Input: part model. Units: mm. Frame: model coordinates. A direction names the side the tool comes from. Round coordinates to 2 decimals unless told otherwise and drop trailing zeros. Loops run counter-clockwise (first coordinate to the right, second up) from the corner with the lowest first, then second, coordinate; pieces in that order, holes last. Notation, with made-up numbers: (89, 26.5) - (142, 26.5) arc R15 cw to (142, 32.5) - close; hole circle Ø7 at (61, 61). An arc over 180 degrees is marked (long way). Write each question's results on one line, items separated by ' | '.
from build123d import *

# Parameters (mm, degrees)
BOSS_EXTRUDE1_DEPTH     = 3
CUT_EXTRUDE1_DEPTH      = 5
CUT_EXTRUDE1_DEPTH_BACK = 3
SKETCH2_W               = 111
SKETCH2_H               = 61


with BuildPart() as part:
    # Sketch1 → Boss-Extrude1 (new body)
    with BuildSketch(Plane(origin=(0, 0, 0), x_dir=(1, 0, 0), z_dir=(0, 1, 0))):
        with BuildLine():
            Line((-75.361284995, 38.602305476), (85.638715005, 38.602305476))
            ThreePointArc((85.638715005, 38.602305476), (89.174248911, 37.137839381), (90.638715005, 33.602305476))
            Line((90.638715005, 33.602305476), (90.638715005, -36.397694524))
            ThreePointArc((90.638715005, -36.397694524), (89.174248911, -39.93322843), (85.638715005, -41.397694524))
            Line((85.638715005, -41.397694524), (-75.361284995, -41.397694524))
            ThreePointArc((-75.361284995, -41.397694524), (-78.896818901, -39.93322843), (-80.361284995, -36.397694524))
            Line((-80.361284995, -36.397694524), (-80.361284995, 33.602305476))
            ThreePointArc((-80.361284995, 33.602305476), (-78.896818901, 37.137839381), (-75.361284995, 38.602305476))
        make_face()
    extrude(amount=BOSS_EXTRUDE1_DEPTH)

    # Sketch2 → Cut-Extrude1 (cut, two sides: drawn at the far end of the back side and taken through both)
    with BuildSketch(Plane(origin=(0, 0, 0), x_dir=(1, 0, 0), z_dir=(0, 1, 0)).offset(-CUT_EXTRUDE1_DEPTH_BACK)):
        with Locations((5.138715005, -1.994135041)):
            Rectangle(SKETCH2_W, SKETCH2_H)
    extrude(amount=CUT_EXTRUDE1_DEPTH + CUT_EXTRUDE1_DEPTH_BACK, mode=Mode.SUBTRACT)


solid = part.part
1. Section query C-C, the plane x = 33. Output: boundary loops of the cut face in (y, z).
Answer:
outline: (0, -38.6) - (3, -38.6) - (3, -28.51) - (0, -28.51) - close; (0, 32.49) - (3, 32.49) - (3, 41.4) - (0, 41.4) - close
2. Contact query for a flat-ended pin moving along its axis: pin 1 (2 mm diameter, centred on x = -48.5, z = -23.5, fed in from +Y). Output: stop coordinate, or through.
Answer:
pin 1: through
3. Line query: line 1 (X direction, y = 2.35, z = -23); line 2 (Z direction, x = 21, y = 2.5). Output: solid intervals per line, ascending. Write a range as [from, to].
Answer:
line 1: [-80.36, -50.36], [60.64, 90.64] | line 2: [-38.6, -28.51], [32.49, 41.4]
4. Set-up query: faces 5 (the flat face through (60.639, 1, 2)), 6 (the flat face through (-80.361, 1, 2)). Return all of +Z, -Z, +X, -X, +Y, -Y with unobstructed straight access to the full face (end or side cutting, diameter ignored); none if empty.
Answer:
face 5: +Y, -Y | face 6: +Z, -Z, -X, +Y, -Y
5. Section query B-B, the plane y = 1.9. Output: boundary loops of the cut face in (x, z).
Answer:
outline: (-80.36, -33.6) arc R5 ccw to (-75.36, -38.6) - (85.64, -38.6) arc R5 ccw to (90.64, -33.6) - (90.64, 36.4) arc R5 ccw to (85.64, 41.4) - (-75.36, 41.4) arc R5 ccw to (-80.36, 36.4) - close; hole (-50.36, -28.51) - (60.64, -28.51) - (60.64, 32.49) - (-50.36, 32.49) - close
6. Mould query, pull axis Z, two halves, no side actions, for faces 1 (the flat face through (6, 3, -35)), 2 (the cylindrical face through (89.213, 1.479, 39.894)), 3 (the flat face through (4, 1, -28.506)), 4 (the flat face through (4, 1, -38.602)). Classes: pulls with the +Z half, pulls with the -Z half, needs draft (parallel to the pull), parting line crosses it, or undercut.
Answer:
face 1: needs draft | face 2: pulls with the +Z half | face 3: undercut | face 4: pulls with the -Z half
7. Section query A-A, the plane z = 20. Output: boundary loops of the cut face in (x, y).
Answer:
outline: (-80.36, 0) - (-50.36, 0) - (-50.36, 3) - (-80.36, 3) - close; (60.64, 0) - (90.64, 0) - (90.64, 3) - (60.64, 3) - close
